from build123d import *

# Parameters (mm, degrees)
EXTRUDE_1_DEPTH     = 37
EXTRUDE_2_DEPTH     = 3
CUT_EXTRUDE_1_DEPTH = 191.257719948
CUT_EXTRUDE_2_DEPTH = 189.833259782


with BuildPart() as part:
    # 草图1 → 凸台-拉伸1 (new body)
    with BuildSketch(Plane.XY):
        Polygon((0, 3), (-48.301428863, 3), (-77, 50.830951895), (-77, 170), (-80, 170), (-80, 50), (-50, 0), (0, 0), align=None)
    extrude(amount=EXTRUDE_1_DEPTH)

    # 草图3 → 凸台-拉伸2 (add)
    with BuildSketch(Plane(origin=(0, 0, 0), x_dir=(-1, 0, 0), z_dir=(0, 0, -1))):
        Polygon((77, 170), (58, 170), (0, 22), (0, 3), (48.301428863, 3), (77, 50.830951895), align=None)
    extrude(amount=-EXTRUDE_2_DEPTH)

    # 草图4 → 切除-拉伸1 (cut, through all)
    with BuildSketch(Plane(origin=(-77, 0, 0), x_dir=(0, 0, -1), z_dir=(1, 0, 0))):
        with BuildLine():
            Line((-14.4, 155), (-14.4, 145))
            ThreePointArc((-14.4, 145), (-18.5, 140.9), (-22.6, 145))
            Line((-22.6, 145), (-22.6, 155))
            ThreePointArc((-22.6, 155), (-18.5, 159.1), (-14.4, 155))
        make_face()
        with BuildLine():
            Line((-14.4, 107), (-14.4, 75))
            ThreePointArc((-14.4, 75), (-18.5, 70.9), (-22.6, 75))
            Line((-22.6, 75), (-22.6, 107))
            ThreePointArc((-22.6, 107), (-18.5, 111.1), (-14.4, 107))
        make_face()
    extrude(amount=-CUT_EXTRUDE_1_DEPTH, mode=Mode.SUBTRACT)

    # 草图5 → 切除-拉伸2 (cut, through all)
    with BuildSketch(Plane(origin=(0, 3, 0), x_dir=(1, 0, 0), z_dir=(0, 1, 0))):
        with BuildLine():
            Line((-22, -22.6), (-32, -22.6))
            ThreePointArc((-32, -22.6), (-36.1, -18.5), (-32, -14.4))
            Line((-32, -14.4), (-22, -14.4))
            ThreePointArc((-22, -14.4), (-17.9, -18.5), (-22, -22.6))
        make_face()
    extrude(amount=-CUT_EXTRUDE_2_DEPTH, mode=Mode.SUBTRACT)


solid = part.part
Can you work these out from the model? Positions are in its coordinate system, mm. A direction names the side the tool comes from. Give positions to 0.01 mm unless a question says otherwise; leave off trailing zeros. Order: outer loops, then holes, each group sorted by start corner. A loop starts at its lowest first (then second) coordinate and runs counter-clockwise, first axis right, second up. Notation, with made-up numbers: M 52.5,8.5 L 98.5,8.5 A21 ccw 98.5,22.5 Z; hole C -29,17 d4. An arc over 180 degrees is marked long. Use one line per item in the form item = value. Start each with the question number.
Item 1: If I drill on line 1 along X through (y, z) = (152, 5); line 2 along Y through (x, z) = (-35.5, 29.5), over which ranges is the centre line in solid material (lowest first)?
Item 2: If we section it at C-C (z = 29.5): Write out the boundary of the cut face in (x, y), then the cut area to 3 significant figures.
Item 3: If we section it at D-D (x = -13): Write out the boundary of the cut face in (y, z), then the cut area to 3 significant figures.
Item 4: For faces 1 (the flat face through (-29.406, 97.036, 1.479)), 2 (the flat face through (-27, 2, 14.4)), 3 (the flat face through (-24, 3, 24)), 4 (the flat face through (-78, 150, 14.4)), which set-ups out of +Z, -Z, +X, -X, +Y, -Y let a thin tool reach every point of the face, with its end or its side?
Item 5: We'd pull the mould along Y, two halves only. Please class faces 5 (the flat face through (-62.45, 26.58, 19.76)), 6 (the flat face through (-78, 91, 22.6)), 7 (the cylindrical face through (-78.5, 140.9, 18.4)), 8 (the flat face through (-79, 79, 37)): +Y half, -Y half, draft (parallel to the pull), parting line (faces both ways), or undercut.
Item 6: If we section it at B-B (y = 95.5): Write out the boundary of the cut face in (x, z).
Item 7: If we section it at A-A (z = 18.5): Write out the boundary of the cut face in (x, y).
Item 8: Will these pins go through, and if not, where does the flat tip stop? pin 1 Ø1 at (y, z) = (39, 24.5) entering from +X; pin 2 Ø1.5 at (x, y) = (-78.5, 85.5) entering from -Z; pin 3 Ø1 at (y, z) = (91.5, 26) entering from +X; pin 4 Ø6 at (x, z) = (-55.5, 26.5) entering from +Y.
Outcome:
q1.line_1 = -80 to -77
q1.line_2 = 0 to 3
q2.outline = M -80,50 L -50,0 L 0,0 L 0,3 L -48.3,3 L -77,50.83 L -77,170 L -80,170 Z
q2.area = 677 mm2
q3.outline = M 0,0 L 55.17,0 L 55.17,3 L 3,3 L 3,37 L 0,37 Z
q3.area = 268 mm2
q4.face_1 = +Z, -Z, +X, +Y
q4.face_2 = +Y, -Y
q4.face_3 = +Z, +X, +Y
q4.face_4 = +X, -X
q5.face_5 = +Y half
q5.face_6 = undercut
q5.face_7 = undercut
q5.face_8 = draft
q6.outline = M -80,0 L -28.8,0 L -28.8,3 L -77,3 L -77,14.4 L -80,14.4 Z; M -80,22.6 L -77,22.6 L -77,37 L -80,37 Z
q7.outline = M -80,50 L -50,0 L -36.1,0 L -36.1,3 L -48.3,3 L -77,50.83 L -77,70.9 L -80,70.9 Z; M -80,111.1 L -77,111.1 L -77,140.9 L -80,140.9 Z; M -80,159.1 L -77,159.1 L -77,170 L -80,170 Z; M -17.9,0 L 0,0 L 0,3 L -17.9,3 Z
q8.pin_1 = -69.6
q8.pin_2 = 0
q8.pin_3 = -77
q8.pin_4 = 20
